Read the model definition and answer for the solid it produces. Units are mm, in the model's axes. Round coordinates to 2 decimals unless told otherwise and drop trailing zeros. Order: outer loops, then holes, each group sorted by start corner. A loop starts at its lowest first (then second) coordinate and runs counter-clockwise, first axis right, second up.
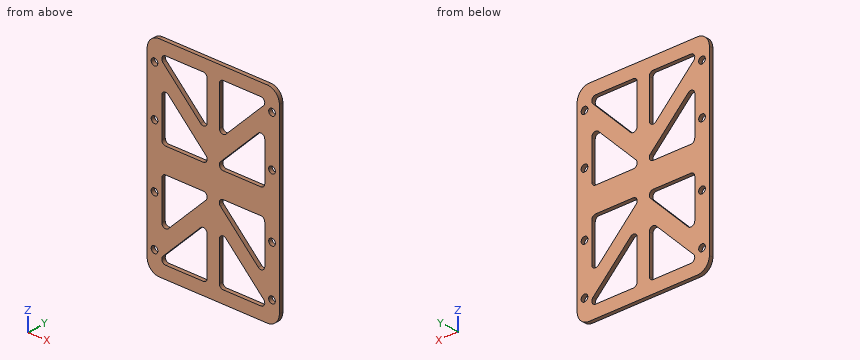
from build123d import *

# Parameters (mm, degrees)
BOSS_EXTRUDE1_DEPTH  = 3.175
M5_CLEARANCE_HOLE1_D = 5.5
CUT_EXTRUDE1_DEPTH   = 99.833045415


with BuildPart() as part:
    # Sketch1 → Boss-Extrude1 (new body)
    with BuildSketch(Plane(origin=(0, 0, 0), x_dir=(1, 0, 0), z_dir=(0, 1, 0))):
        with BuildLine():
            Line((-44.329, -82.5), (44.329, -82.5))
            ThreePointArc((44.329, -82.5), (51.400067812, -79.571067812), (54.329, -72.5))
            Line((54.329, -72.5), (54.329, 72.5))
            ThreePointArc((54.329, 72.5), (51.400067812, 79.571067812), (44.329, 82.5))
            Line((44.329, 82.5), (-44.329, 82.5))
            ThreePointArc((-44.329, 82.5), (-51.400067812, 79.571067812), (-54.329, 72.5))
            Line((-54.329, 72.5), (-54.329, -72.5))
            ThreePointArc((-54.329, -72.5), (-51.400067812, -79.571067812), (-44.329, -82.5))
        make_face()
    extrude(amount=BOSS_EXTRUDE1_DEPTH)

    # M5 Clearance Hole1 (through all)
    with Locations(Plane(origin=(0, 3.175, 0), x_dir=(1, 0, 0), z_dir=(0, 1, 0))):
        with Locations((-48.29, 65), (-48.29, -65), (48.29, -65), (48.29, 65), (-48.29, 25), (-48.29, -25), (48.29, 25), (48.29, -25)):
            Hole(M5_CLEARANCE_HOLE1_D / 2)

    # Sketch4 → Cut-Extrude1 (cut, through all)
    with BuildSketch(Plane(origin=(0, 3.175, 0), x_dir=(1, 0, 0), z_dir=(0, 1, 0))):
        with BuildLine():
            Line((-42.329, 44.154), (-42.329, 13.175))
            ThreePointArc((-42.329, 13.175), (-41.39906403, 10.92993597), (-39.154, 10))
            Line((-39.154, 10), (-8.175, 10))
            ThreePointArc((-8.175, 10), (-5.241682484, 11.959980102), (-5.92993597, 15.42006403))
            Line((-5.92993597, 15.42006403), (-36.90893597, 46.39906403))
            ThreePointArc((-36.90893597, 46.39906403), (-40.369019898, 47.087317516), (-42.329, 44.154))
        make_face()
        with BuildLine():
            Line((39.154, 72.5), (8.175, 72.5))
            ThreePointArc((8.175, 72.5), (5.92993597, 71.57006403), (5, 69.325))
            Line((5, 69.325), (5, 38.346))
            ThreePointArc((5, 38.346), (6.959980102, 35.412682484), (10.42006403, 36.10093597))
            Line((10.42006403, 36.10093597), (41.39906403, 67.07993597))
            ThreePointArc((41.39906403, 67.07993597), (42.087317516, 70.540019898), (39.154, 72.5))
        make_face()
        with BuildLine():
            Line((-5, 69.325), (-5, 38.346))
            ThreePointArc((-5, 38.346), (-6.959980102, 35.412682484), (-10.42006403, 36.10093597))
            Line((-10.42006403, 36.10093597), (-41.39906403, 67.07993597))
            ThreePointArc((-41.39906403, 67.07993597), (-42.087317516, 70.540019898), (-39.154, 72.5))
            Line((-39.154, 72.5), (-8.175, 72.5))
            ThreePointArc((-8.175, 72.5), (-5.92993597, 71.57006403), (-5, 69.325))
        make_face()
        with BuildLine():
            Line((5.92993597, 15.42006403), (36.90893597, 46.39906403))
            ThreePointArc((36.90893597, 46.39906403), (40.369019898, 47.087317516), (42.329, 44.154))
            Line((42.329, 44.154), (42.329, 13.175))
            ThreePointArc((42.329, 13.175), (41.39906403, 10.92993597), (39.154, 10))
            Line((39.154, 10), (8.175, 10))
            ThreePointArc((8.175, 10), (5.241682484, 11.959980102), (5.92993597, 15.42006403))
        make_face()
        with BuildLine():
            Line((42.329, -44.154), (42.329, -13.175))
            ThreePointArc((42.329, -13.175), (41.39906403, -10.92993597), (39.154, -10))
            Line((39.154, -10), (8.175, -10))
            ThreePointArc((8.175, -10), (5.241682484, -11.959980102), (5.92993597, -15.42006403))
            Line((5.92993597, -15.42006403), (36.90893597, -46.39906403))
            ThreePointArc((36.90893597, -46.39906403), (40.369019898, -47.087317516), (42.329, -44.154))
        make_face()
        with BuildLine():
            Line((5, -69.325), (5, -38.346))
            ThreePointArc((5, -38.346), (6.959980102, -35.412682484), (10.42006403, -36.10093597))
            Line((10.42006403, -36.10093597), (41.39906403, -67.07993597))
            ThreePointArc((41.39906403, -67.07993597), (42.087317516, -70.540019898), (39.154, -72.5))
            Line((39.154, -72.5), (8.175, -72.5))
            ThreePointArc((8.175, -72.5), (5.92993597, -71.57006403), (5, -69.325))
        make_face()
        with BuildLine():
            Line((-39.154, -72.5), (-8.175, -72.5))
            ThreePointArc((-8.175, -72.5), (-5.92993597, -71.57006403), (-5, -69.325))
            Line((-5, -69.325), (-5, -38.346))
            ThreePointArc((-5, -38.346), (-6.959980102, -35.412682484), (-10.42006403, -36.10093597))
            Line((-10.42006403, -36.10093597), (-41.39906403, -67.07993597))
            ThreePointArc((-41.39906403, -67.07993597), (-42.087317516, -70.540019898), (-39.154, -72.5))
        make_face()
        with BuildLine():
            Line((-5.92993597, -15.42006403), (-36.90893597, -46.39906403))
            ThreePointArc((-36.90893597, -46.39906403), (-40.369019898, -47.087317516), (-42.329, -44.154))
            Line((-42.329, -44.154), (-42.329, -13.175))
            ThreePointArc((-42.329, -13.175), (-41.39906403, -10.92993597), (-39.154, -10))
            Line((-39.154, -10), (-8.175, -10))
            ThreePointArc((-8.175, -10), (-5.241682484, -11.959980102), (-5.92993597, -15.42006403))
        make_face()
    extrude(amount=-CUT_EXTRUDE1_DEPTH, mode=Mode.SUBTRACT)


solid = part.part
Q1. A cutting plane is placed at C-C, the plane y = 1.8. Give the number of separate pieces and of enclosed holes in the cut face, plus the area to 3 significant figures.
Outcome:
separate pieces: 1
enclosed holes: 16
area: 10,900 mm2
Q2. A cutting plane is placed at B-B, the plane z = 25. Give the vertices of the cut face in (x, y) (3 decimals), plus the area to 3 significant figures.
Outcome:
outline: (-54.329, 0) - (-51.04, 0) - (-51.04, 3.175) - (-54.329, 3.175) - close; (-45.54, 0) - (-42.329, 0) - (-42.329, 3.175) - (-45.54, 3.175) - close; (-15.51, 0) - (15.51, 0) - (15.51, 3.175) - (-15.51, 3.175) - close; (42.329, 0) - (45.54, 0) - (45.54, 3.175) - (42.329, 3.175) - close; (51.04, 0) - (54.329, 0) - (54.329, 3.175) - (51.04, 3.175) - close
area: 140 mm2
Q3. A cutting plane is placed at A-A, the plane x = -48.29. Give the vertices of the cut face in (y, z) (3 decimals).
Outcome:
outline: (0, -81.682) - (3.175, -81.682) - (3.175, -67.75) - (0, -67.75) - close; (0, -62.25) - (3.175, -62.25) - (3.175, -27.75) - (0, -27.75) - close; (0, -22.25) - (3.175, -22.25) - (3.175, 22.25) - (0, 22.25) - close; (0, 27.75) - (3.175, 27.75) - (3.175, 62.25) - (0, 62.25) - close; (0, 67.75) - (3.175, 67.75) - (3.175, 81.682) - (0, 81.682) - close
Q4. Straight lines are drawn through the part: probe 1 along Z at (x, y) = (-41, 2.2); probe 2 along Z at (x, y) = (-48.29, 1.5); probe 3 along X at (y, z) = (1.6, 25). For each, find the intervals that lie inside material, in ascending order.
Outcome:
probe 1: z = -82.5 to -71.91, -66.68 to -46.74, -10.59 to 10.59, 46.74 to 66.68, 71.91 to 82.5
probe 2: z = -81.68 to -67.75, -62.25 to -27.75, -22.25 to 22.25, 27.75 to 62.25, 67.75 to 81.68
probe 3: x = -54.33 to -51.04, -45.54 to -42.33, -15.51 to 15.51, 42.33 to 45.54, 51.04 to 54.33
